The listing builds one solid part. Answer for the finished solid, in the listing's coordinates (mm). A direction names the side the tool comes from. Give positions to 0.01 mm unless a question says otherwise; leave off trailing zeros. Write each loop counter-clockwise with the first axis right and the second up, starting at its lowest first coordinate (ties: lowest second). Pieces come first, ordered by that corner, then holes. Notation, with made-up numbers: M 43.25,31.5 L 77.25,31.5 A29 cw 77.25,54.5 Z; hole C 23.5,85.25 d5. An arc over 180 degrees is marked long. Return JSON: item names as keys, results as strings.
from build123d import *

# Parameters (mm, degrees)
SKETCH1_W           = 114.3
SKETCH1_H           = 114.3
SKETCH1_W_2         = 38.1
SKETCH1_H_2         = 38.1
BOSS_EXTRUDE1_DEPTH = 76.2
SKETCH3_W           = 76.2
SKETCH3_H           = 76.2
CUT_EXTRUDE2_DEPTH  = 54.61
SKETCH5_W           = 114.3
SKETCH5_H           = 114.3
SKETCH5_W_2         = 76.2
SKETCH5_H_2         = 76.2
CUT_EXTRUDE3_DEPTH  = 12.7
CHAMFER1_SIZE       = 12.7
CUT_EXTRUDE4_REACH  = 144.699
SKETCH6_W           = 76.2
SKETCH6_H           = 41.91
SKETCH7_R           = 6.35
CUT_EXTRUDE5_DEPTH  = 5.08
SKETCH9_R           = 6.35
CUT_EXTRUDE6_DEPTH  = 5.08
CUT_EXTRUDE7_START  = -5.08
SKETCH8_R           = 6.35
CUT_EXTRUDE7_DEPTH  = 5.08


with BuildPart() as part:
    # Sketch1 → Boss-Extrude1 (new body)
    with BuildSketch(Plane(origin=(0, 0, 0), x_dir=(1, 0, 0), z_dir=(0, 1, 0))):
        Rectangle(SKETCH1_W, SKETCH1_H)
        Rectangle(SKETCH1_W_2, SKETCH1_H_2, mode=Mode.SUBTRACT)
    extrude(amount=BOSS_EXTRUDE1_DEPTH)

    # Sketch3 → Cut-Extrude2 (cut)
    with BuildSketch(Plane(origin=(0, 76.2, 0), x_dir=(1, 0, 0), z_dir=(0, 1, 0))):
        Rectangle(SKETCH3_W, SKETCH3_H)
    extrude(amount=-CUT_EXTRUDE2_DEPTH, mode=Mode.SUBTRACT)

    # Sketch5 → Cut-Extrude3 (cut)
    with BuildSketch(Plane(origin=(0, 76.2, 0), x_dir=(1, 0, 0), z_dir=(0, 1, 0))):
        Rectangle(SKETCH5_W, SKETCH5_H)
        Rectangle(SKETCH5_W_2, SKETCH5_H_2, mode=Mode.SUBTRACT)
    extrude(amount=-CUT_EXTRUDE3_DEPTH, mode=Mode.SUBTRACT)

    # Chamfer1
    chamfer1_edges = [part.edges().sort_by_distance(p)[0] for p in [
        (57.15, 31.75, 57.15),
        (-57.15, 31.75, 57.15),
        (-57.15, 31.75, -57.15),
        (57.15, 31.75, -57.15),
    ]]
    chamfer(chamfer1_edges, length=CHAMFER1_SIZE)

    # Sketch6 → Cut-Extrude4 (cut, up to next)
    with BuildSketch(Plane.XY.offset(57.15), mode=Mode.PRIVATE) as cut_extrude4_sk1:
        with Locations((0, 42.545)):
            Rectangle(SKETCH6_W, SKETCH6_H)
    cut_extrude4_tool1 = extrude(cut_extrude4_sk1.sketch, amount=-CUT_EXTRUDE4_REACH, mode=Mode.PRIVATE) & part.part
    add(cut_extrude4_tool1.solids().sort_by_distance((0, 42.545, 57.15))[0], mode=Mode.SUBTRACT)

    # Sketch7 → Cut-Extrude5 (cut)
    with BuildSketch(Plane(origin=(0, 21.59, 0), x_dir=(1, 0, 0), z_dir=(0, 1, 0))):
        with Locations(Location((0, -47.625, 0), (0, 0, 270))):
            Circle(SKETCH7_R)
    extrude(amount=-CUT_EXTRUDE5_DEPTH, mode=Mode.SUBTRACT)

    # Sketch9 → Cut-Extrude6 (cut)
    with BuildSketch(Plane.ZY.offset(-38.1)):
        with Locations((47.625, 42.545)):
            Circle(SKETCH9_R)
    extrude(amount=-CUT_EXTRUDE6_DEPTH, mode=Mode.SUBTRACT)

    # Sketch8 → Cut-Extrude7 (cut)
    with BuildSketch(Plane(origin=(-38.1, 0, 0), x_dir=(0, 0, -1), z_dir=(1, 0, 0)).offset(CUT_EXTRUDE7_START)):
        with Locations(Location((-47.625, 42.545, 0), (0, 0, 180))):
            Circle(SKETCH8_R)
    extrude(amount=CUT_EXTRUDE7_DEPTH, mode=Mode.SUBTRACT)


solid = part.part
Item 1: A cutting plane is placed at C-C, the plane y = 33. Write down the section's boundary in (x, z), plus the area to 3 significant figures.
Geometry results:
{"outline": "M -57.15,-44.45 L -44.45,-57.15 L 44.45,-57.15 L 57.15,-44.45 L 57.15,44.45 L 44.45,57.15 L 38.1,57.15 L 38.1,-38.1 L -38.1,-38.1 L -38.1,57.15 L -44.45,57.15 L -57.15,44.45 Z", "area": "5,480 mm2"}
Item 2: A cutting plane is placed at A-A, the plane z = 6.5. Write down the section's boundary in (x, y).
Geometry results:
{"outline": "M -57.15,0 L -19.05,0 L -19.05,21.59 L -38.1,21.59 L -38.1,63.5 L -57.15,63.5 Z; M 19.05,0 L 57.15,0 L 57.15,63.5 L 38.1,63.5 L 38.1,21.59 L 19.05,21.59 Z"}
Item 3: A cutting plane is placed at B-B, the plane x = 16. Write down the section's boundary in (y, z).
Geometry results:
{"outline": "M 0,-57.15 L 63.5,-57.15 L 63.5,-38.1 L 21.59,-38.1 L 21.59,-19.05 L 0,-19.05 Z; M 0,19.05 L 21.59,19.05 L 21.59,57.15 L 0,57.15 Z"}
Item 4: Find the intervals of material crossed by line 1 (X direction, y = 24.5, z = -7); line 2 (Z direction, x = 1, y = 17); line 3 (X direction, y = 12.5, z = -19), in increasing order.
Geometry results:
{"line 1": "x = -57.15 to -38.1, 38.1 to 57.15", "line 2": "z = -57.15 to -19.05, 19.05 to 41.35, 53.9 to 57.15", "line 3": "x = -57.15 to -19.05, 19.05 to 57.15"}
Item 5: A cutting plane is placed at D-D, the plane y = 20. Write down the section's boundary in (x, z) (3 decimals).
Geometry results:
{"outline": "M -57.15,-44.45 L -44.45,-57.15 L 44.45,-57.15 L 57.15,-44.45 L 57.15,44.45 L 44.45,57.15 L -44.45,57.15 L -57.15,44.45 Z; hole M -19.05,-19.05 L 19.05,-19.05 L 19.05,19.05 L -19.05,19.05 Z; hole C 0,47.625 d12.7"}
Item 6: Given pin 1 Ø4 at (y, z) = (44, 47.5) entering from -X; pin 2 Ø2 at (x, z) = (-18, 33.5) entering from +Y, each flat-ended and moving along its own axis, determine where each tip first touches the part or whether it passes through.
Geometry results:
{"pin 1": "stops at x = -56.1", "pin 2": "stops at y = 21.59"}
Item 7: Which of the six approach directions +Z, -Z, +X, -X, +Y, -Y give full straight-line access (tool end or side, diameter ignored) to faces 4 (the flat face through (0, 11, 19.05)), 5 (the cylindrical face through (0.28, 19.09, 41.28)), 6 (the flat face through (-1, 31, -57.15)), 7 (the flat face through (43.18, 43, 48)), 8 (the flat face through (-1, 43, -38.1))?
Geometry results:
{"face 4": "+Y, -Y", "face 5": "+Y", "face 6": "-Z, +X, -X, +Y, -Y", "face 7": "none", "face 8": "+Z, +Y"}
Item 8: Determine the mould class of faces 1 (the flat face through (50.9, 31.3, -50.7)), 2 (the flat face through (-43.18, 42, 48)), 3 (the flat face through (50.9, 31.3, 50.7)) for opening direction Z: +Z half, -Z half, draft (parallel to the pull), parting line (faces both ways), or undercut.
Geometry results:
{"face 1": "-Z half", "face 2": "undercut", "face 3": "+Z half"}
